Verification items for the finished model (mm, model axes). Face numbers are marked on the shaded views. A direction names the side the tool comes from. Give positions to 0.01 mm unless a question says otherwise; leave off trailing zeros. Loops run counter-clockwise (first coordinate to the right, second up) from the corner with the lowest first, then second, coordinate; pieces in that order, holes last. Notation, with made-up numbers: M 77,-10.5 L 84,-10.5 A22 cw 84,18.5 Z; hole C -10.75,87 d8. An arc over 180 degrees is marked long. Put each result on its own line as item: value. Start each with the question number.
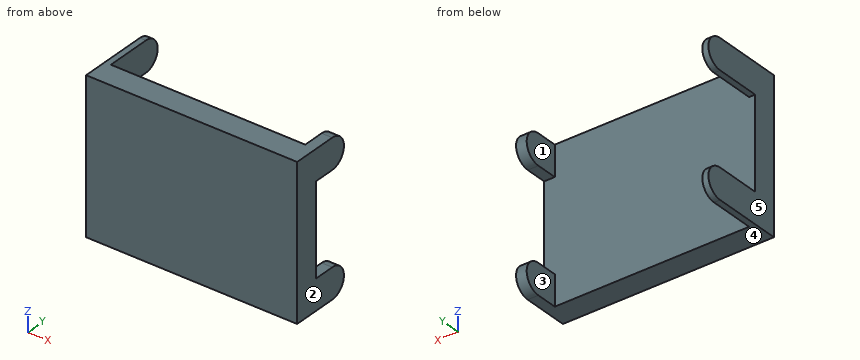
from build123d import *

# Parameters (mm, degrees)
SKETCH1_W           = 34.75
SKETCH1_H           = 25
BOSS_EXTRUDE1_DEPTH = 4
SKETCH2_W           = 1.75
SKETCH2_H           = 5
BOSS_EXTRUDE2_DEPTH = 6
SKETCH4_W           = 1
SKETCH4_H           = 5
BOSS_EXTRUDE3_DEPTH = 10
FILLET2_RADIUS      = 2.5
FILLET2_LENGTH      = 1
FILLET3_RADIUS      = 2.5
FILLET3_LENGTH      = 1
FILLET4_RADIUS      = 2.5
FILLET4_LENGTH      = 1.75
FILLET5_RADIUS      = 2.5
FILLET5_LENGTH      = 1.75


with BuildPart() as part:
    # Sketch1 → Boss-Extrude1 (new body)
    with BuildSketch(Plane(origin=(0, 0, 0), x_dir=(1, 0, 0), z_dir=(0, 1, 0))):
        Rectangle(SKETCH1_W, SKETCH1_H)
    extrude(amount=BOSS_EXTRUDE1_DEPTH)

    # Sketch2 → Boss-Extrude2 (add)
    with BuildSketch(Plane(origin=(0, 4, 0), x_dir=(1, 0, 0), z_dir=(0, 1, 0))):
        with Locations((16.5, -10)):
            Rectangle(SKETCH2_W, SKETCH2_H)
        with Locations((16.5, 10)):
            Rectangle(SKETCH2_W, SKETCH2_H)
    extrude(amount=BOSS_EXTRUDE2_DEPTH)

    # Sketch4 → Boss-Extrude3 (add)
    with BuildSketch(Plane(origin=(0, 4, 0), x_dir=(1, 0, 0), z_dir=(0, 1, 0))):
        with Locations((-16.875, 10)):
            Rectangle(SKETCH4_W, SKETCH4_H)
        with Locations((-16.875, -10)):
            Rectangle(SKETCH4_W, SKETCH4_H)
    extrude(amount=BOSS_EXTRUDE3_DEPTH)

    # Fillet2: full round fillet: the end face becomes a half cylinder, R = half its width
    fillet2_face = Plane((-16.875, 14, -10), x_dir=(1, 0, 0), z_dir=(0, 1, 0))  # on the end face: x along it, z out of the body
    fillet2_slab = fillet2_face.offset(-FILLET2_RADIUS / 2) * Box(FILLET2_LENGTH, 2 * FILLET2_RADIUS, FILLET2_RADIUS, mode=Mode.PRIVATE)  # the body's end, R deep
    fillet2_round = Plane((-16.875, 11.5, -10), x_dir=(0, 1, 0), z_dir=(1, 0, 0)) * Cylinder(FILLET2_RADIUS, FILLET2_LENGTH, mode=Mode.PRIVATE)  # its axis R under the face
    add(fillet2_slab - fillet2_round, mode=Mode.SUBTRACT)

    # Fillet3: full round fillet: the end face becomes a half cylinder, R = half its width
    fillet3_face = Plane((-16.875, 14, 10), x_dir=(1, 0, 0), z_dir=(0, 1, 0))  # on the end face: x along it, z out of the body
    fillet3_slab = fillet3_face.offset(-FILLET3_RADIUS / 2) * Box(FILLET3_LENGTH, 2 * FILLET3_RADIUS, FILLET3_RADIUS, mode=Mode.PRIVATE)  # the body's end, R deep
    fillet3_round = Plane((-16.875, 11.5, 10), x_dir=(0, 1, 0), z_dir=(1, 0, 0)) * Cylinder(FILLET3_RADIUS, FILLET3_LENGTH, mode=Mode.PRIVATE)  # its axis R under the face
    add(fillet3_slab - fillet3_round, mode=Mode.SUBTRACT)

    # Fillet4: full round fillet: the end face becomes a half cylinder, R = half its width
    fillet4_face = Plane((16.5, 10, -10), x_dir=(1, 0, 0), z_dir=(0, 1, 0))  # on the end face: x along it, z out of the body
    fillet4_slab = fillet4_face.offset(-FILLET4_RADIUS / 2) * Box(FILLET4_LENGTH, 2 * FILLET4_RADIUS, FILLET4_RADIUS, mode=Mode.PRIVATE)  # the body's end, R deep
    fillet4_round = Plane((16.5, 7.5, -10), x_dir=(0, 1, 0), z_dir=(1, 0, 0)) * Cylinder(FILLET4_RADIUS, FILLET4_LENGTH, mode=Mode.PRIVATE)  # its axis R under the face
    add(fillet4_slab - fillet4_round, mode=Mode.SUBTRACT)

    # Fillet5: full round fillet: the end face becomes a half cylinder, R = half its width
    fillet5_face = Plane((16.5, 10, 10), x_dir=(1, 0, 0), z_dir=(0, 1, 0))  # on the end face: x along it, z out of the body
    fillet5_slab = fillet5_face.offset(-FILLET5_RADIUS / 2) * Box(FILLET5_LENGTH, 2 * FILLET5_RADIUS, FILLET5_RADIUS, mode=Mode.PRIVATE)  # the body's end, R deep
    fillet5_round = Plane((16.5, 7.5, 10), x_dir=(0, 1, 0), z_dir=(1, 0, 0)) * Cylinder(FILLET5_RADIUS, FILLET5_LENGTH, mode=Mode.PRIVATE)  # its axis R under the face
    add(fillet5_slab - fillet5_round, mode=Mode.SUBTRACT)


solid = part.part
Q1. Cross-section at B-B, the plane y = 6.75. Record the boundary of the cut face in (x, z) (3 decimals), then the cut area to 3 significant figures.
Q2. Cross-section at D-D, the plane x = -0.5. Record the boundary of the cut face in (y, z), then the cut area to 3 significant figures.
Q3. Cross-section at C-C, the plane z = -10. Record the boundary of the cut face in (x, y) (3 decimals).
Q4. Scan lines: L1, parallel to Y at x = -1.5, z = 0; L2, parallel to X at y = 13, z = -10.25 (3 decimals); L3, parallel to X at y = 6.5, z = 8.5 (3 decimals). Record each from-to range of solid material in increasing order.
Q5. Release check for a two-part mould opening along X. For the marked faces 3, 4 and 5 record: pulls with the +X half, pulls with the -X half, needs draft (parallel to the pull), parting line crosses it, or undercut.
Q6. Go/stop test with flat-tipped pins: pin 1 (12.5 mm diameter, centred on x = 0.5, z = -2, fed in from +Y); pin 2 (1.5 mm diameter, centred on x = 3, y = 5, fed in from -Z). Record where each tip stops, or that it passes through.
Q7. Cross-section at A-A, the plane y = 13. Record the boundary of the cut face in (x, z) (3 decimals).
Q8. Set-up check for the marked faces 1 and 2: record each of +Z, -Z, +X, -X, +Y, -Y from which the full face is reachable in a straight line by a thin tool's end or side.
Ans:
1. outline: M -17.375,-12.5 L -16.375,-12.5 L -16.375,-7.5 L -17.375,-7.5 Z; M -17.375,7.5 L -16.375,7.5 L -16.375,12.5 L -17.375,12.5 Z; M 15.625,-12.5 L 17.375,-12.5 L 17.375,-7.5 L 15.625,-7.5 Z; M 15.625,7.5 L 17.375,7.5 L 17.375,12.5 L 15.625,12.5 Z
1. area: 27.5 mm^2
2. outline: M 0,-12.5 L 4,-12.5 L 4,12.5 L 0,12.5 Z
2. area: 100 mm^2
3. outline: M -17.375,0 L 17.375,0 L 17.375,10 L 15.625,10 L 15.625,4 L -16.375,4 L -16.375,14 L -17.375,14 Z
4. L1: y = 0 to 4
4. L2: x = -17.375 to -16.375
4. L3: x = -17.375 to -16.375, 15.625 to 17.375
5. face 3: undercut
5. face 4: needs draft
5. face 5: pulls with the -X half
6. pin 1: stops at y = 4
6. pin 2: passes through
7. outline: M -17.375,-12 L -16.375,-12 L -16.375,-8 L -17.375,-8 Z; M -17.375,8 L -16.375,8 L -16.375,12 L -17.375,12 Z
8. face 1: +Z, -Z, +Y
8. face 2: +Z, -Z, +X, +Y, -Y
